Here's how the part is built. I have some questions about the finished solid (model axes, mm). Face numbers are marked on the shaded views. A direction names the side the tool comes from. Coordinates: 2 decimals unless noted, no trailing zeros. Loops run counter-clockwise (first coordinate to the right, second up) from the corner with the lowest first, then second, coordinate; pieces in that order, holes last. Notation, with made-up numbers: M 28.25,52.25 L 84.25,52.25 A14 ccw 84.25,57.25 Z; hole C 86.5,89.5 d8. An arc over 180 degrees is marked long. Use CSV: the item, a comma, the result in double quotes. Start each with the question number.
Q1. Which directions (+Z, -Z, +X, -X, +Y, -Y) give clear straight access to the entire face, cutting with the end or side of a thin tool? Please do the marked faces 1 and 2.
Q2. If we section it at C-C (y = -6): Please give me the cut outline in (x, z), and give its area (3 significant figures).
Q3. Please list where these lines run through material, in increasing order: probe 1 along Y at (x, z) = (0, -2.4); probe 2 along Y at (x, z) = (0, -0.8); probe 3 along Z at (x, y) = (3.5, -3). Write a range as [from, to].
Q4. If we section it at A-A (x = 0): Please give me the cut outline in (y, z).
Q5. For pin 1 Ø3 at (y, z) = (2.5, 1.5) entering from +X; pin 2 Ø2 at (x, z) = (6, 0) entering from +Y; pin 3 Ø4.5 at (x, y) = (1.5, 0) entering from +Z; pin 4 Ø4 at (x, y) = (-0.5, 0) entering from +Z, each with a flat end and sliding along its axis, tell me the tip position at first contact or that it passes through.
Q6. If we section it at D-D (x = -3.75): Please give me the cut outline in (y, z), and give its area (3 significant figures).
Q7. If we mould it in two halves opening along X, with no side actions, what happens to the marked faces 3, 4, 5 and 6? For each: +X half, -X half, draft (parallel to the pull), parting line (faces both ways), or undercut.
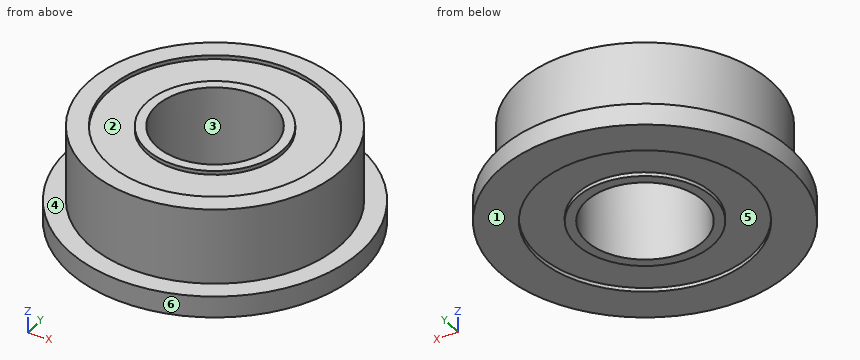
from build123d import *

# Parameters (mm, degrees)
SKETCH_1_R          = 6.5
EXTRUDE_1_DEPTH     = 2.5
SKETCH_4_R          = 7.5
EXTRUDE_2_DEPTH     = 1.1
SKETCH_2_R          = 3
CUT_EXTRUDE_1_DEPTH = 6
SKETCH_3_R          = 5.5
SKETCH_3_R_2        = 3.5
CUT_EXTRUDE_2_DEPTH = 0.2


with BuildPart() as part:
    # 草圖1 → 填料-伸長1 (new body, symmetric)
    with BuildSketch(Plane.XY):
        Circle(SKETCH_1_R)
    extrude(amount=EXTRUDE_1_DEPTH, both=True)

    # 草圖4 → 填料-伸長2 (add)
    with BuildSketch(Plane(origin=(0, 0, -2.5), x_dir=(-1, 0, 0), z_dir=(0, 0, -1))):
        Circle(SKETCH_4_R)
    extrude(amount=-EXTRUDE_2_DEPTH)

    # 草圖2 → 除料-伸長1 (cut, through all)
    with BuildSketch(Plane.XY.offset(2.5)):
        Circle(SKETCH_2_R)
    extrude(amount=-CUT_EXTRUDE_1_DEPTH, mode=Mode.SUBTRACT)

    # 草圖3 → 除料-伸長2 (cut)
    with BuildSketch(Plane.XY.offset(2.5)):
        Circle(SKETCH_3_R)
        Circle(SKETCH_3_R_2, mode=Mode.SUBTRACT)
    cut_extrude_2 = extrude(amount=-CUT_EXTRUDE_2_DEPTH, mode=Mode.SUBTRACT)

    # 鏡射1: 除料-伸長2 across plane
    add(cut_extrude_2.mirror(Plane.XY), mode=Mode.SUBTRACT)


solid = part.part
Results below:
1,face 1,"-Z, +X, -X, +Y, -Y"
1,face 2,"+Z"
2,outline,"M -4.5,-2.5 L 4.5,-2.5 L 4.5,-1.4 L 2.5,-1.4 L 2.5,2.5 L -2.5,2.5 L -2.5,-1.4 L -4.5,-1.4 Z"
2,area,"29.4 mm^2"
3,probe 1,"[-7.5, -5.5], [-3.5, -3], [3, 3.5], [5.5, 7.5]"
3,probe 2,"[-6.5, -3], [3, 6.5]"
3,probe 3,"[-2.3, 2.3]"
4,outline,"M -7.5,-2.5 L -5.5,-2.5 L -5.5,-2.3 L -3.5,-2.3 L -3.5,-2.5 L -3,-2.5 L -3,2.5 L -3.5,2.5 L -3.5,2.3 L -5.5,2.3 L -5.5,2.5 L -6.5,2.5 L -6.5,-1.4 L -7.5,-1.4 Z; M 3,-2.5 L 3.5,-2.5 L 3.5,-2.3 L 5.5,-2.3 L 5.5,-2.5 L 7.5,-2.5 L 7.5,-1.4 L 6.5,-1.4 L 6.5,2.5 L 5.5,2.5 L 5.5,2.3 L 3.5,2.3 L 3.5,2.5 L 3,2.5 Z"
5,pin 1,"x = 6.42"
5,pin 2,"y = 4.15"
5,pin 3,"z = 2.5"
5,pin 4,"through"
6,outline,"M -6.5,-2.5 L -4.02,-2.5 L -4.02,-2.3 L 4.02,-2.3 L 4.02,-2.5 L 6.5,-2.5 L 6.5,-1.4 L 5.31,-1.4 L 5.31,2.5 L 4.02,2.5 L 4.02,2.3 L -4.02,2.3 L -4.02,2.5 L -5.31,2.5 L -5.31,-1.4 L -6.5,-1.4 Z"
6,area,"52.5 mm^2"
7,face 3,"undercut"
7,face 4,"draft"
7,face 5,"undercut"
7,face 6,"parting line"
